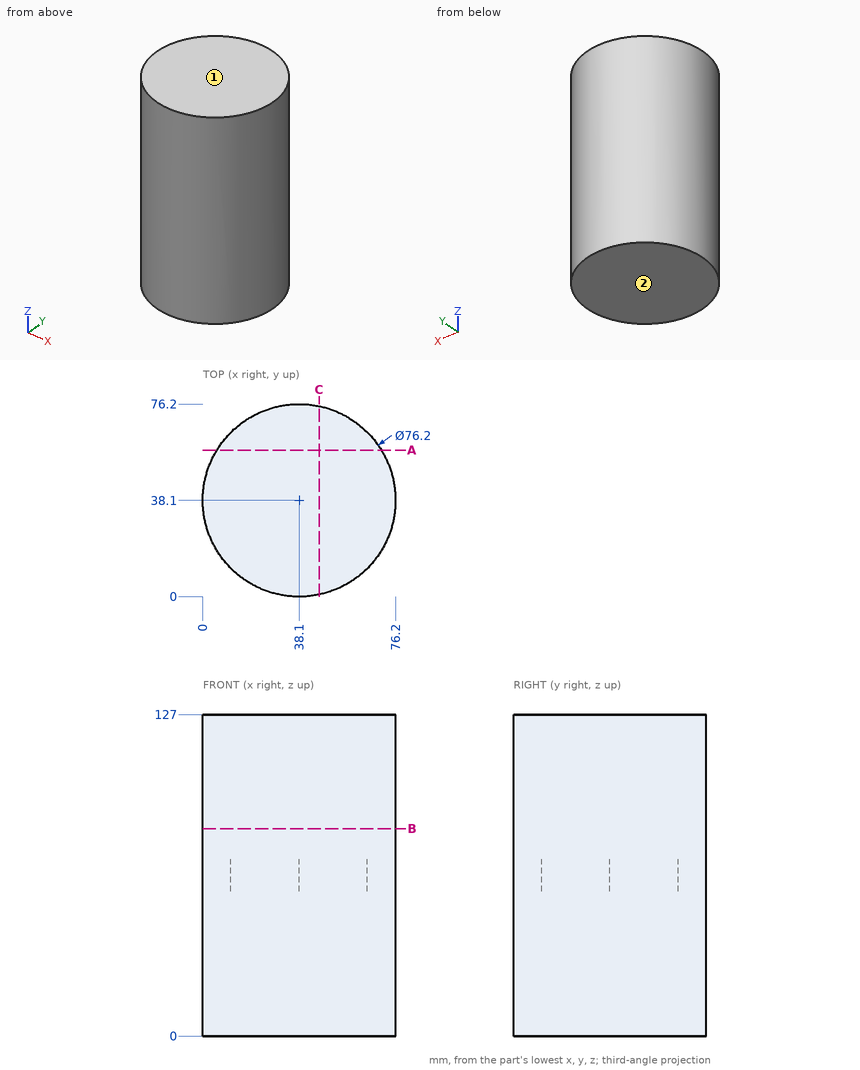
Verification items for this drawing (mm, ordinates from the low corner). Coordinates: 2 decimals unless noted, no trailing zeros. Loops run counter-clockwise (first coordinate to the right, second up) from the corner with the lowest first, then second, coordinate; pieces in that order, holes last. Notation, with made-up numbers: (88, 23) - (141, 23) arc R11 ccw to (141, 31) - close; hole circle Ø2 at (-38.75, 10.25). An arc over 180 degrees is marked (long way). Use one line per item in the form item = value. Start each with the question number.
Item 1: Mould release check, pull along Z, two halves, no side actions. Record for the marked faces 1 and 2: +Z half, -Z half, draft (parallel to the pull), parting line (faces both ways), or undercut.
Item 2: Thickness scan on probe 1 along X at (y, z) = (60.5, 119.5); probe 2 along Y at (x, z) = (15.5, 37); probe 3 along X at (y, z) = (55, 63). Record the ranges inside material, lowest first.
Item 3: Gauge pin test, flat ends, axial feed: pin 1 (12 mm diameter, centred on x = 50.5, z = 80.5, fed in from -Y); pin 2 (8 mm diameter, centred on y = 33, z = 91.5, fed in from +X); pin 3 (12 mm diameter, centred on y = 21.5, z = 22.5, fed in from -X). Record the tip position at first contact, or that the pin passes through.
Item 4: Section check A-A, the plane y = 58. Enter the section's corners in (x, z), and give its area (3 significant figures).
Item 5: Section check C-C, the plane x = 46. Enter the section's corners in (y, z).
Item 6: Section check B-B, the plane z = 82. Enter the section's corners in (x, y), and give its area (3 significant figures).
Computed:
q1.face_1 = +Z half
q1.face_2 = -Z half
q2.probe_1 = 7.28 to 68.92
q2.probe_2 = 7.43 to 68.77
q2.probe_3 = 3.95 to 72.25
q3.pin_1 = 0.54
q3.pin_2 = 76.18
q3.pin_3 = 1.5
q4.outline = (5.61, 0) - (70.59, 0) - (70.59, 127) - (5.61, 127) - close
q4.area = 8,250 mm2
q5.outline = (0.83, 0) - (75.37, 0) - (75.37, 127) - (0.83, 127) - close
q6.outline = circle Ø76.2 at (38.1, 38.1)
q6.area = 4,560 mm2
